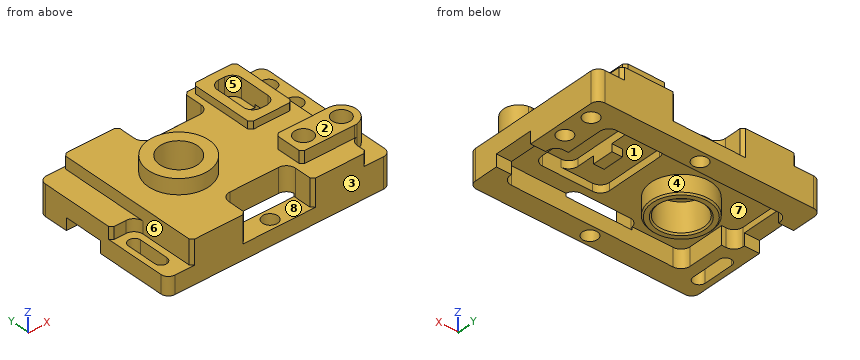
from build123d import *

# Parameters (mm, degrees)
SKETCH_1_W                  = 148
SKETCH_1_H                  = 98
EXTRUDE_1_DEPTH             = 28
FILLET_1_R                  = 5
SKETCH_3_W                  = 110
SKETCH_3_H                  = 70
CUT_EXTRUDE_1_DEPTH         = 12
FILLET_2_R                  = 6
CUT_EXTRUDE_2_DEPTH         = 5
CUT_EXTRUDE_3_DEPTH         = 5
SKETCH_7_W                  = 7
SKETCH_7_H                  = 14
EXTRUDE_2_DEPTH             = 5
SKETCH_8_R                  = 20
EXTRUDE_3_DEPTH             = 12
SKETCH_9_R                  = 15
CUT_EXTRUDE_4_DEPTH         = 20
SKETCH_10_W                 = 10
SKETCH_10_H                 = 26
CUT_EXTRUDE_5_DEPTH         = 8
CUT_EXTRUDE_6_DEPTH         = 18
CUT_EXTRUDE_7_DEPTH         = 8
SKETCH_14_W                 = 16
SKETCH_14_H                 = 98
CUT_EXTRUDE_8_DEPTH         = 8
CUT_EXTRUDE_9_DEPTH         = 8
CHAMFER_1_SIZE              = 2
EXTRUDE_START               = 10
SKETCH_17_R                 = 20
EXTRUDE_4_DEPTH             = 10
CHAMFER_2_SIZE              = 1
SKETCH_18_R                 = 12.5
CUT_EXTRUDE_10_DEPTH        = 97.545326143
SKETCH_19_W                 = 28
SKETCH_19_H                 = 44
EXTRUDE_5_DEPTH             = 5
SKETCH_20_W                 = 16
SKETCH_20_H                 = 32
CUT_EXTRUDE_11_DEPTH        = 13
FILLET_3_R                  = 6
CHAMFER_3_SIZE              = 2
EXTRUDE_START_2             = 8
EXTRUDE_6_DEPTH             = 8
CHAMFER_4_SIZE              = 2
CUT_EXTRUDE_12_DEPTH        = 97.545326143
SKETCH_23_R                 = 5
CUT_EXTRUDE_13_DEPTH        = 97.545326143
HOLE_WIZARD_12_0_12_1_D     = 12
HOLE_WIZARD_12_0_12_1_DEPTH = 10
HOLE_WIZARD_12_0_12_1_TIP   = 3.605163714
SKETCH_26_R                 = 5
CUT_EXTRUDE_14_DEPTH        = 91.978019323


with BuildPart() as part:
    # 草图1 → 凸台-拉伸1 (new body)
    with BuildSketch(Plane.XY):
        Rectangle(SKETCH_1_W, SKETCH_1_H)
    extrude(amount=EXTRUDE_1_DEPTH)

    # 圆角1
    fillet_1_edges = [part.edges().sort_by_distance(p)[0] for p in [
        (-74, 49, 14),
        (74, 49, 14),
        (74, -49, 14),
        (-74, -49, 14),
    ]]
    fillet(fillet_1_edges, radius=FILLET_1_R)

    # 草图3 → 切除-拉伸1 (cut)
    with BuildSketch(Plane(origin=(0, 0, 0), x_dir=(-1, 0, 0), z_dir=(0, 0, -1))):
        with BuildLine():
            Line((-58, -35), (-55, -35))
            Line((-55, -35), (-55, 5))
            Line((-55, 5), (-58, 5))
            ThreePointArc((-58, 5), (-62.242640687, 3.242640687), (-64, -1))
            Line((-64, -1), (-64, -29))
            ThreePointArc((-64, -29), (-62.242640687, -33.242640687), (-58, -35))
        make_face()
        Rectangle(SKETCH_3_W, SKETCH_3_H)
        with BuildLine():
            Line((55, 35), (55, -5))
            Line((55, -5), (58, -5))
            ThreePointArc((58, -5), (62.242640687, -3.242640687), (64, 1))
            Line((64, 1), (64, 29))
            ThreePointArc((64, 29), (62.242640687, 33.242640687), (58, 35))
            Line((58, 35), (55, 35))
        make_face()
    extrude(amount=-CUT_EXTRUDE_1_DEPTH, mode=Mode.SUBTRACT)

    # 圆角2
    fillet_2_edges = [part.edges().sort_by_distance(p)[0] for p in [
        (55, 35, 6),
        (-55, -35, 6),
    ]]
    fillet(fillet_2_edges, radius=FILLET_2_R)

    # 草图4 → 切除-拉伸2 (cut)
    with BuildSketch(Plane(origin=(0, 0, 12), x_dir=(-1, 0, 0), z_dir=(0, 0, -1))):
        with BuildLine():
            Line((-46, -25), (-13, -25))
            ThreePointArc((-13, -25), (-8.757359313, -23.242640687), (-7, -19))
            Line((-7, -19), (-7, 19))
            ThreePointArc((-7, 19), (-8.757359313, 23.242640687), (-13, 25))
            Line((-13, 25), (-46, 25))
            ThreePointArc((-46, 25), (-50.242640687, 23.242640687), (-52, 19))
            Line((-52, 19), (-52, -19))
            ThreePointArc((-52, -19), (-50.242640687, -23.242640687), (-46, -25))
        make_face()
    extrude(amount=-CUT_EXTRUDE_2_DEPTH, mode=Mode.SUBTRACT)

    # 草图6 → 切除-拉伸3 (cut)
    with BuildSketch(Plane(origin=(0, 0, 17), x_dir=(-1, 0, 0), z_dir=(0, 0, -1))):
        with BuildLine():
            Line((-46, -25), (-34, -25))
            ThreePointArc((-34, -25), (-29.757359313, -23.242640687), (-28, -19))
            Line((-28, -19), (-28, 19))
            ThreePointArc((-28, 19), (-29.757359313, 23.242640687), (-34, 25))
            Line((-34, 25), (-46, 25))
            ThreePointArc((-46, 25), (-50.242640687, 23.242640687), (-52, 19))
            Line((-52, 19), (-52, -19))
            ThreePointArc((-52, -19), (-50.242640687, -23.242640687), (-46, -25))
        make_face()
    extrude(amount=-CUT_EXTRUDE_3_DEPTH, mode=Mode.SUBTRACT)

    # 草图7 → 凸台-拉伸2 (add)
    with BuildSketch(Plane(origin=(0, 0, 17), x_dir=(-1, 0, 0), z_dir=(0, 0, -1))):
        with Locations((-24.5, 0)):
            Rectangle(SKETCH_7_W, SKETCH_7_H)
    extrude(amount=EXTRUDE_2_DEPTH)

    # 草图8 → 凸台-拉伸3 (add)
    with BuildSketch(Plane(origin=(0, 0, 12), x_dir=(-1, 0, 0), z_dir=(0, 0, -1))):
        with Locations((24, 0)):
            Circle(SKETCH_8_R)
    extrude(amount=EXTRUDE_3_DEPTH)

    # 草图9 → 切除-拉伸4 (cut)
    with BuildSketch(Plane(origin=(0, 0, 0), x_dir=(-1, 0, 0), z_dir=(0, 0, -1))):
        with Locations((24, 0)):
            Circle(SKETCH_9_R)
    extrude(amount=-CUT_EXTRUDE_4_DEPTH, mode=Mode.SUBTRACT)

    # 草图10 → 切除-拉伸5 (cut)
    with BuildSketch(Plane(origin=(0, 0, 0), x_dir=(-1, 0, 0), z_dir=(0, 0, -1))):
        with Locations((-69, -15)):
            Rectangle(SKETCH_10_W, SKETCH_10_H)
        with Locations((69, 15)):
            Rectangle(SKETCH_10_W, SKETCH_10_H)
    extrude(amount=-CUT_EXTRUDE_5_DEPTH, mode=Mode.SUBTRACT)

    # 草图12 → 切除-拉伸6 (cut)
    with BuildSketch(Plane.XY.offset(28)):
        with BuildLine():
            Line((22, -49), (-22, -49))
            Line((-22, -49), (-22, -36))
            ThreePointArc((-22, -36), (-20.242640687, -31.757359313), (-16, -30))
            Line((-16, -30), (16, -30))
            ThreePointArc((16, -30), (20.242640687, -31.757359313), (22, -36))
            Line((22, -36), (22, -49))
        make_face()
        with BuildLine():
            Line((-22, 49), (-22, 36))
            ThreePointArc((-22, 36), (-20.242640687, 31.757359313), (-16, 30))
            Line((-16, 30), (16, 30))
            ThreePointArc((16, 30), (20.242640687, 31.757359313), (22, 36))
            Line((22, 36), (22, 49))
            Line((22, 49), (-22, 49))
        make_face()
    extrude(amount=-CUT_EXTRUDE_6_DEPTH, mode=Mode.SUBTRACT)

    # 草图13 → 切除-拉伸7 (cut)
    with BuildSketch(Plane.XY.offset(28)):
        with BuildLine():
            Line((74, -49), (58, -49))
            Line((58, -49), (58, -41.716233646))
            ThreePointArc((58, -41.716233646), (59.376689498, -37.89196901), (62.875, -35.822646028))
            ThreePointArc((62.875, -35.822646028), (71, -26), (62.875, -16.177353972))
            ThreePointArc((62.875, -16.177353972), (59.376689498, -14.10803099), (58, -10.283766354))
            Line((58, -10.283766354), (58, 49))
            Line((58, 49), (74, 49))
            Line((74, 49), (74, -49))
        make_face()
    extrude(amount=-CUT_EXTRUDE_7_DEPTH, mode=Mode.SUBTRACT)

    # 草图14 → 切除-拉伸8 (cut)
    with BuildSketch(Plane.XY.offset(28)):
        with Locations((-66, 0)):
            Rectangle(SKETCH_14_W, SKETCH_14_H)
    extrude(amount=-CUT_EXTRUDE_8_DEPTH, mode=Mode.SUBTRACT)

    # 草图15 → 切除-拉伸9 (cut)
    with BuildSketch(Plane.XY.offset(20)):
        with BuildLine():
            Line((-58, -49), (-74, -49))
            Line((-74, -49), (-74, -6))
            Line((-74, -6), (-64, -6))
            ThreePointArc((-64, -6), (-59.757359313, -7.757359313), (-58, -12))
            Line((-58, -12), (-58, -49))
        make_face()
    extrude(amount=-CUT_EXTRUDE_9_DEPTH, mode=Mode.SUBTRACT)

    # 倒角1
    chamfer_1_edges = [part.edges().sort_by_distance(p)[0] for p in [
        (22, -49, 19),
        (-22, -49, 19),
        (-22, 49, 19),
        (22, 49, 19),
        (58, 49, 24),
        (58, -49, 24),
        (-58, 49, 24),
        (-58, -49, 20),
        (-74, -6, 16),
    ]]
    chamfer(chamfer_1_edges, length=CHAMFER_1_SIZE)

    # 草图17 → 凸台-拉伸4 (add)
    with BuildSketch(Plane.XY.offset(28).offset(EXTRUDE_START)):
        with Locations(Location((-24, 0, 0), (0, 0, 180))):
            Circle(SKETCH_17_R)
    extrude(amount=-EXTRUDE_4_DEPTH)

    # 倒角2
    chamfer_2_edges = [part.edges().sort_by_distance(p)[0] for p in [
        (-4, 0, 0),
        (-9, 0, 0),
    ]]
    chamfer(chamfer_2_edges, length=CHAMFER_2_SIZE)

    # 草图18 → 切除-拉伸10 (cut, through all)
    with BuildSketch(Plane.XY.offset(38)):
        with Locations((-24, 0)):
            Circle(SKETCH_18_R)
    extrude(amount=-CUT_EXTRUDE_10_DEPTH, mode=Mode.SUBTRACT)

    # 草图19 → 凸台-拉伸5 (add)
    with BuildSketch(Plane.XY.offset(28)):
        with Locations((40, 25)):
            Rectangle(SKETCH_19_W, SKETCH_19_H)
    extrude(amount=EXTRUDE_5_DEPTH)

    # 草图20 → 切除-拉伸11 (cut)
    with BuildSketch(Plane.XY.offset(33)):
        with Locations((40, 25)):
            Rectangle(SKETCH_20_W, SKETCH_20_H)
    extrude(amount=-CUT_EXTRUDE_11_DEPTH, mode=Mode.SUBTRACT)

    # 圆角3
    fillet_3_edges = [part.edges().sort_by_distance(p)[0] for p in [
        (32, 9, 27.5),
        (48, 41, 26.5),
        (32, 41, 26.5),
        (48, 9, 27.5),
    ]]
    fillet(fillet_3_edges, radius=FILLET_3_R)

    # 倒角3
    chamfer_3_edges = [part.edges().sort_by_distance(p)[0] for p in [
        (54, 3, 30.5),
        (54, 47, 30.5),
        (26, 47, 30.5),
        (26, 3, 30.5),
    ]]
    chamfer(chamfer_3_edges, length=CHAMFER_3_SIZE)

    # 草图21 → 凸台-拉伸6 (add)
    with BuildSketch(Plane.XY.offset(28).offset(EXTRUDE_START_2)):
        with BuildLine():
            Line((26, -16), (26, -36))
            Line((26, -36), (61, -36))
            ThreePointArc((61, -36), (61.941684585, -35.955562774), (62.875, -35.822646028))
            ThreePointArc((62.875, -35.822646028), (71, -26), (62.875, -16.177353972))
            ThreePointArc((62.875, -16.177353972), (61.941684585, -16.044437226), (61, -16))
            Line((61, -16), (26, -16))
        make_face()
    extrude(amount=-EXTRUDE_6_DEPTH)

    # 倒角4
    chamfer_4_edges = [part.edges().sort_by_distance(p)[0] for p in [
        (26, -16, 32),
        (26, -36, 32),
    ]]
    chamfer(chamfer_4_edges, length=CHAMFER_4_SIZE)

    # 草图22 → 切除-拉伸12 (cut, through all)
    with BuildSketch(Plane(origin=(0, 0, 0), x_dir=(-1, 0, 0), z_dir=(0, 0, -1))):
        with BuildLine():
            Line((62.19694392, -35), (62.19694392, -15))
            ThreePointArc((62.19694392, -15), (66.19694392, -11), (70.19694392, -15))
            Line((70.19694392, -15), (70.19694392, -35))
            ThreePointArc((70.19694392, -35), (66.19694392, -39), (62.19694392, -35))
        make_face()
    extrude(amount=-CUT_EXTRUDE_12_DEPTH, mode=Mode.SUBTRACT)

    # 草图23 → 切除-拉伸13 (cut, through all)
    with BuildSketch(Plane(origin=(0, 0, 0), x_dir=(-1, 0, 0), z_dir=(0, 0, -1))):
        with Locations((0, 42)):
            Circle(SKETCH_23_R)
        with Locations((0, -42)):
            Circle(SKETCH_23_R)
    extrude(amount=-CUT_EXTRUDE_13_DEPTH, mode=Mode.SUBTRACT)

    # Ø12.0 (12) 直径孔1
    with Locations(Plane(origin=(61, -26, 36), x_dir=(1, 0, 0), z_dir=(0, 0, 1))):
        with Locations((0, 0), (-25, 0)):
            Hole(HOLE_WIZARD_12_0_12_1_D / 2, depth=HOLE_WIZARD_12_0_12_1_DEPTH)
            with Locations((0, 0, -(HOLE_WIZARD_12_0_12_1_DEPTH + HOLE_WIZARD_12_0_12_1_TIP / 2))):  # 118° drill point
                Cone(0, HOLE_WIZARD_12_0_12_1_D / 2, HOLE_WIZARD_12_0_12_1_TIP, mode=Mode.SUBTRACT)

    # 草图26 → 切除-拉伸14 (cut, through all)
    with BuildSketch(Plane.XY.offset(20)):
        with Locations((66.01411415, 35)):
            Circle(SKETCH_26_R)
        with Locations((66.01411415, 15)):
            Circle(SKETCH_26_R)
    extrude(amount=-CUT_EXTRUDE_14_DEPTH, mode=Mode.SUBTRACT)


solid = part.part
Here's how the part is built. I have some questions about the finished solid (model axes, mm). Face numbers are marked on the shaded views. A direction names the side the tool comes from. Round coordinates to 2 decimals unless told otherwise and drop trailing zeros. Write each loop counter-clockwise with the first axis right and the second up, starting at its lowest first coordinate (ties: lowest second). Pieces come first, ordered by that corner, then holes.
1. If we mould it in two halves opening along Y, with no side actions, what happens to the marked faces 1, 2, 3 and 4? For each: released by +Y, released by -Y, zero draft, split by the parting line, or undercut.
2. Suppose I cut it at C-C (z = 4). State how many separate pieces and enclosed holes the cut face has, and give its area (3 significant figures).
3. Will these pins go through, and if not, where does the flat tip stop? pin 1 Ø8 at (x, y) = (70.5, -18) entering from -Z; pin 2 Ø5 at (x, y) = (-50, 7) entering from -Z; pin 3 Ø7 at (x, y) = (-1.5, -43.5) entering from +Z.
4. For the marked faces 5, 6, 7 and 8, which set-ups out of +Z, -Z, +X, -X, +Y, -Y let a thin tool reach every point of the face, with its end or its side?
5. Suppose I cut it at B-B (x = 0). List the corners of the cut face in (y, z) for me.
6. I need wall thicknesses on L1, parallel to Y at x = 0, z = 6; L2, parallel to X at y = 35.5, z = 14; L3, parallel to X at y = 38, z = 19.5. Which ranges of each line are inside material? Lowest first, please.
7. Suppose I cut it at A-A (z = 31.5). List the corners of the cut face in (x, y) for me (3 decimals), and give its area (3 significant figures).
Answer sheet:
1. face 1: undercut
1. face 2: zero draft
1. face 3: released by -Y
1. face 4: undercut
2. separate pieces: 3
2. enclosed holes: 6
2. area: 5,610 mm2
3. pin 1: stops at z = 8
3. pin 2: stops at z = 12
3. pin 3: stops at z = 10
4. face 5: +Z
4. face 6: +Z, -X, -Y
4. face 7: -Z
4. face 8: +Z, -Y
5. outline: (-49, 0) - (-47, 0) - (-47, 10) - (-49, 10) - close; (-37, 0) - (-35, 0) - (-35, 10) - (-37, 10) - close; (-30, 12) - (30, 12) - (30, 28) - (-30, 28) - close; (35, 0) - (37, 0) - (37, 10) - (35, 10) - close; (47, 0) - (49, 0) - (49, 10) - (47, 10) - close
6. L1: y = -49 to -47, -37 to -35, 35 to 37, 47 to 49
6. L2: x = -74 to -21.98, 21.98 to 61.04, 70.99 to 74
6. L3: x = -74 to -22, 22 to 62.01, 70.01 to 74
7. outline: circle Ø40 at (-24, 0); (26, -34) - (28, -36) - (61, -36) arc R10 ccw to (61, -16) - (28, -16) - (26, -18) - close; (26, 5) - (28, 3) - (52, 3) - (54, 5) - (54, 45) - (52, 47) - (28, 47) - (26, 45) - close; hole circle Ø25 at (-24, 0); hole circle Ø12 at (36, -26); hole (32, 15) arc R6 ccw to (38, 9) - (42, 9) arc R6 ccw to (48, 15) - (48, 35) arc R6 ccw to (42, 41) - (38, 41) arc R6 ccw to (32, 35) - close; hole circle Ø12 at (61, -26)
7. area: 2,140 mm2
